For this review, take the finished solid that the model builds, in its own axes (mm). Face numbers are marked on the shaded views. A direction names the side the tool comes from. Coordinates: 2 decimals unless noted, no trailing zeros. Loops run counter-clockwise (first coordinate to the right, second up) from the corner with the lowest first, then second, coordinate; pieces in that order, holes last. Notation, with made-up numbers: M 27,78.25 L 63,78.25 A29 cw 63,114.25 Z; hole C 36,35.5 d4. An arc over 180 degrees is marked long. Use one line per item in the form item = value.
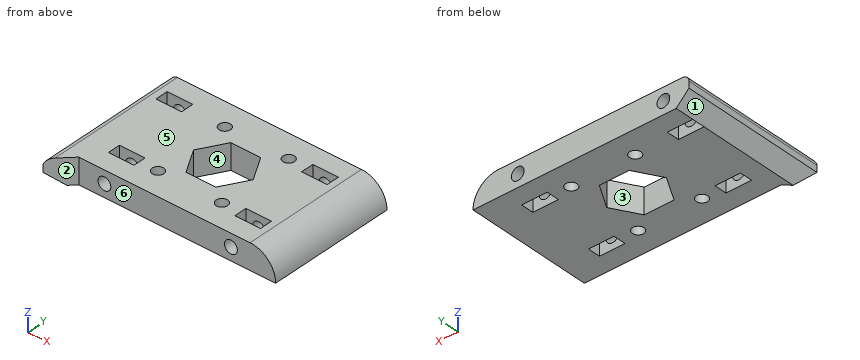
```python
from build123d import *

# Parameters (mm, degrees)
SKETCH1_W           = 4
SKETCH1_H           = 2
SKETCH1_R           = 0.9
BOSS_EXTRUDE1_DEPTH = 4
SKETCH3_R           = 1
CUT_EXTRUDE1_DEPTH  = 20
SKETCH3_3_R         = 1
CUT_EXTRUDE2_DEPTH  = 10
SKETCH5_R           = 1
CUT_EXTRUDE3_DEPTH  = 10
CHAMFER2_SIZE       = 2
FILLET2_R           = 1
FILLET3_R           = 4


with BuildPart() as part:
    # Sketch1 → Boss-Extrude1 (new body)
    # profile 1 of 2: a face of its own
    with BuildSketch(Plane.XY):
        Polygon((-9.335901083, -15.296943817), (-6.335901083, -15.296943817), (24.464098917, -15.296943817), (24.464098917, 4.703056183), (-9.335901083, 4.703056183), align=None)
        with Locations((-2.335901083, -11.296943817)):
            Rectangle(SKETCH1_W, SKETCH1_H, mode=Mode.SUBTRACT)
        with Locations((2.564098917, -11.296943817)):
            Circle(SKETCH1_R, mode=Mode.SUBTRACT)
        with Locations((12.564098917, -11.296943817)):
            Circle(SKETCH1_R, mode=Mode.SUBTRACT)
        with Locations((17.464098917, -11.296943817)):
            Rectangle(SKETCH1_W, SKETCH1_H, mode=Mode.SUBTRACT)
        with Locations((-5.335901083, 0.703056183)):
            Rectangle(SKETCH1_W, SKETCH1_H, mode=Mode.SUBTRACT)
        with Locations((2.564098917, 0.703056183)):
            Circle(SKETCH1_R, mode=Mode.SUBTRACT)
        Polygon((9.896924586, -1.256371234), (12.229750255, -5.296943817), (9.896924586, -9.337516401), (5.231273248, -9.337516401), (2.898447579, -5.296943817), (5.231273248, -1.256371234), align=None, mode=Mode.SUBTRACT)
        with Locations((12.564098917, 0.703056183)):
            Circle(SKETCH1_R, mode=Mode.SUBTRACT)
        with Locations((17.464098917, 0.703056183)):
            Rectangle(SKETCH1_W, SKETCH1_H, mode=Mode.SUBTRACT)
    # profile 2 of 2: a face of its own
    with BuildSketch(Plane.XY):
        Polygon((-9.335901083, -15.296943817), (-9.335901083, -18.296943817), (-6.335901083, -15.296943817), align=None)
    extrude(amount=BOSS_EXTRUDE1_DEPTH)

    # Sketch3 → Cut-Extrude1 (cut)
    with BuildSketch(Plane.XZ.offset(15.296943817)):
        with Locations((17.464098917, 2)):
            Circle(SKETCH3_R)
    extrude(amount=-CUT_EXTRUDE1_DEPTH, mode=Mode.SUBTRACT)

    # Sketch3<3> → Cut-Extrude2 (cut)
    with BuildSketch(Plane.XZ.offset(15.296943817)):
        with Locations((-2.335901083, 2)):
            Circle(SKETCH3_3_R)
    extrude(amount=-CUT_EXTRUDE2_DEPTH, mode=Mode.SUBTRACT)

    # Sketch5 → Cut-Extrude3 (cut)
    with BuildSketch(Plane(origin=(0, 4.703056183, 0), x_dir=(1, 0, 0), z_dir=(0, 1, 0))):
        with Locations(Location((-5.335901083, -2, 0), (0, 0, 180))):
            Circle(SKETCH5_R)
    extrude(amount=-CUT_EXTRUDE3_DEPTH, mode=Mode.SUBTRACT)

    # Chamfer2
    chamfer2_edges = [part.edges().sort_by_distance(p)[0] for p in [
        (-9.335901083, -6.796943817, 0),
    ]]
    chamfer(chamfer2_edges, length=CHAMFER2_SIZE - 0.0001)  # a hair under: the kernel refuses the full size

    # Fillet2
    fillet2_edges = [part.edges().sort_by_distance(p)[0] for p in [
        (-9.335901083, -6.796943817, 4),
    ]]
    fillet(fillet2_edges, radius=FILLET2_R)

    # Fillet3
    fillet3_edges = [part.edges().sort_by_distance(p)[0] for p in [
        (24.464098917, -5.296943817, 4),
    ]]
    fillet(fillet3_edges, radius=FILLET3_R - 0.0001)  # a hair under: the kernel refuses the full size


solid = part.part
```
1. Consider section A-A on y = -14.5. State how many separate pieces and enclosed holes the cut face has, plus the area to 3 significant figures.
Computed values:
separate_pieces = 1
enclosed_holes = 2
area = 123 mm2
2. Wall thickness on line 1 along X through (y, z) = (0.25, 0.7); line 2 along Y through (x, z) = (-4, 2.2); line 3 along Y through (x, z) = (-4.5, 0.7): over which ranges is each line inside the solid? List them lowest first. Write a range as from..to.
Computed values:
line_1 = -8.04..-7.34, -3.34..1.79, 3.34..11.79, 13.34..15.46, 19.46..24.4
line_2 = -15.3..-12.3, -10.3..-0.3, 1.7..4.7
line_3 = -15.3..-0.3, 1.7..4.7
3. Draft analysis for pull direction Y (two halves, no side actions). For the marked faces 1, 2 and 3, state which applies: +Y half, -Y half, draft (parallel to the pull), parting line (faces both ways), or undercut.
Computed values:
face_1 = draft
face_2 = -Y half
face_3 = undercut
4. Tool access review of the marked faces 4, 5 and 6: name each direction out of +Z, -Z, +X, -X, +Y, -Y from which nothing blocks a thin tool from reaching the whole face with its end or side.
Computed values:
face_4 = +Z, -Z
face_5 = +Z, +X, -X, +Y, -Y
face_6 = +Z, -Z, +X, -Y
5. Consider section D-D on x = 20. Write out the cut boundary in (y, z).
Computed values:
outline = M -15.3,0 L 4.7,0 L 4.7,4 L -15.3,4 Z
6. For pin 1 Ø0.6 at (y, z) = (-11, 2) entering from +X; pin 2 Ø1.2 at (x, z) = (15, 2) entering from -Y; pin 3 Ø1 at (y, z) = (-2.5, 3.5) entering from +X; pin 4 Ø2.5 at (x, y) = (2.56, -11.3) entering from -Z, all flat-tipped, find the tip position at first contact; note any pin that passes through.
Computed values:
pin_1 = 24.08
pin_2 = -15.3
pin_3 = 23.11
pin_4 = 0
